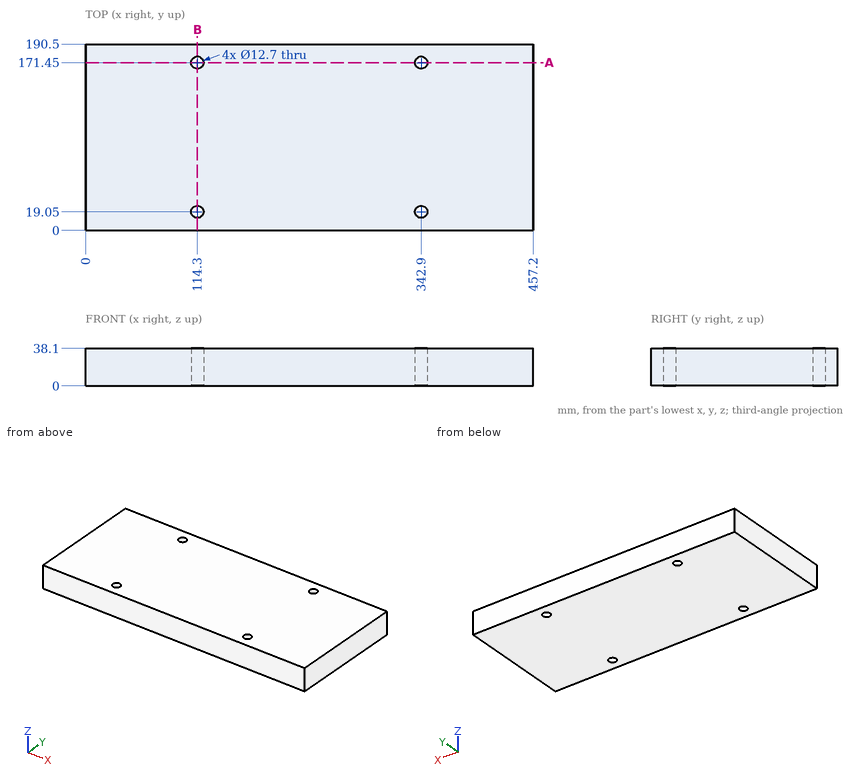
Study the drawing (mm; zero at the part's minimum x, y, z) and answer. Round coordinates to 2 decimals unless told otherwise and drop trailing zeros. Order: outer loops, then holes, each group sorted by start corner. A loop starts at its lowest first (then second) coordinate and runs counter-clockwise, first axis right, second up. Notation, with made-up numbers: M 62,18.25 L 67,18.25 A23 ccw 67,34.25 Z; hole C -2,49 d6. An arc over 180 degrees is marked long. One line per item, written item: value.
Q1. Find section B-B on x = 114.3. Write down the section's boundary in (y, z).
Derived:
outline: M 0,0 L 12.7,0 L 12.7,38.1 L 0,38.1 Z; M 25.4,0 L 165.1,0 L 165.1,38.1 L 25.4,38.1 Z; M 177.8,0 L 190.5,0 L 190.5,38.1 L 177.8,38.1 Z
Q2. Find section A-A on y = 171.45. Write down the section's boundary in (x, z), then the cut area to 3 significant figures.
Derived:
outline: M 0,0 L 107.95,0 L 107.95,38.1 L 0,38.1 Z; M 120.65,0 L 336.55,0 L 336.55,38.1 L 120.65,38.1 Z; M 349.25,0 L 457.2,0 L 457.2,38.1 L 349.25,38.1 Z
area: 16,500 mm²
Q3. Straight lines are drawn through the part: line 1 (Y direction, x = 342, z = 30); line 2 (Y direction, x = 342.9, z = 13.5); line 3 (X direction, y = 171.5, z = 35). For each, find the intervals that lie inside material, in ascending order.
Derived:
line 1: 0 to 12.76, 25.34 to 165.16, 177.74 to 190.5
line 2: 0 to 12.7, 25.4 to 165.1, 177.8 to 190.5
line 3: 0 to 107.95, 120.65 to 336.55, 349.25 to 457.2
